```python
from build123d import *

# Parameters (mm, degrees)
SKETCH1_W               = 50.8
SKETCH1_H               = 50.8
BOSS_EXTRUDE1_DEPTH     = 19.05
F_1_4_CLEARANCE_HOLE1_D = 6.7564
SKETCH9_W               = 12.7
SKETCH9_H               = 50.8
SKETCH9_W_2             = 50.8
SKETCH9_H_2             = 12.7
SKETCH9_W_3             = 31.75
SKETCH9_H_3             = 31.75
CUT_EXTRUDE1_DEPTH      = 12.7


with BuildPart() as part:
    # Sketch1 → Boss-Extrude1 (new body)
    with BuildSketch(Plane(origin=(0, 0, 0), x_dir=(1, 0, 0), z_dir=(0, 1, 0))):
        Rectangle(SKETCH1_W, SKETCH1_H)
    extrude(amount=BOSS_EXTRUDE1_DEPTH)

    # 1/4 Clearance Hole1 (through all)
    with Locations(Plane(origin=(0, 19.05, 0), x_dir=(1, 0, 0), z_dir=(0, 1, 0))):
        with Locations((-19.05, 19.05), (19.05, 19.05), (19.05, -19.05), (-19.05, -19.05)):
            Hole(F_1_4_CLEARANCE_HOLE1_D / 2)

    # Sketch9 → Cut-Extrude1 (cut)
    with BuildSketch(Plane.XZ):
        Rectangle(SKETCH9_W, SKETCH9_H)
        Rectangle(SKETCH9_W_2, SKETCH9_H_2)
        Rectangle(SKETCH9_W_3, SKETCH9_H_3)
    extrude(amount=-CUT_EXTRUDE1_DEPTH, mode=Mode.SUBTRACT)


solid = part.part
```
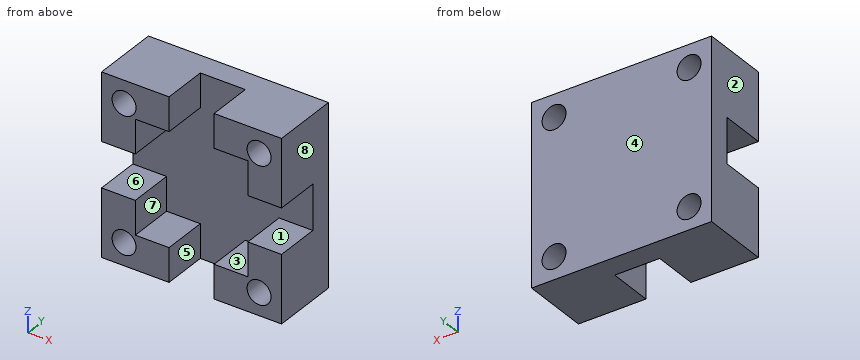
Source: CAD feature listing. Evaluate the final solid. Frame: model axes, mm. Face numbers are marked on the shaded views. A direction names the side the tool comes from. Coordinates: 2 decimals unless noted, no trailing zeros. Write each loop counter-clockwise with the first axis right and the second up, starting at its lowest first coordinate (ties: lowest second). Pieces come first, ordered by that corner, then holes. Notation, with made-up numbers: (16, 86.25) -> (72, 86.25) arc R33 ccw to (72, 117.25) -> close; hole circle Ø11 at (55.5, -7.5). An arc over 180 degrees is marked (long way). Return JSON: item names as keys, results as strings. Group by question number.
1) Ray query, line 1 along X through (y, z) = (10.25, -19.05); line 2 along X through (y, z) = (15, -19.05). Return the intervals inside material, ascending.
2) Section query D-D, the plane z = 8.5. Return loops of the section in (x, y) (3 decimals).
3) Section query C-C, the plane x = -19.05. Return loops of the section in (y, z), plus the area to 3 significant figures.
4) Set-up query: the marked faces 1, 2, 3, 4 and 5. Return all of +Z, -Z, +X, -X, +Y, -Y with unobstructed straight access to the full face (end or side cutting, diameter ignored); none if empty.
5) Section query A-A, the plane y = 7. Return loops of the section in (x, z) (3 decimals), plus the area to 3 significant figures.
6) Contact query for a flat-ended pin moving along its axis: P1, Ø3, axis at x = 16.5, z = 0, coming from the -Y side. Output: stop coordinate, or through.
7) Section query B-B, the plane z = 19.05. Return loops of the section in (x, y).
8) Mould query, pull axis X, two halves, no side actions, for the marked faces 6, 7 and 8. Classes: +X half, -X half, draft (parallel to the pull), parting line (faces both ways), or undercut.
From the geometry:
{
 "1": {"line 1": "-25.4 to -22.43, -15.67 to -6.35, 6.35 to 15.67, 22.43 to 25.4", "line 2": "-25.4 to -22.43, -15.67 to 15.67, 22.43 to 25.4"},
 "2": {"outline": "(-25.4, 0) -> (-15.875, 0) -> (-15.875, 12.7) -> (15.875, 12.7) -> (15.875, 0) -> (25.4, 0) -> (25.4, 19.05) -> (-25.4, 19.05) -> close"},
 "3": {"outline": "(0, -25.4) -> (19.05, -25.4) -> (19.05, -22.43) -> (0, -22.43) -> close; (0, -15.67) -> (19.05, -15.67) -> (19.05, 15.67) -> (0, 15.67) -> (0, 6.35) -> (12.7, 6.35) -> (12.7, -6.35) -> (0, -6.35) -> close; (0, 22.43) -> (19.05, 22.43) -> (19.05, 25.4) -> (0, 25.4) -> close", "area": "549 mm²"},
 "4": {"face 1": "+X, -X, -Y", "face 2": "+Z, -Z, -X, +Y, -Y", "face 3": "-Y", "face 4": "+Z, -Z, +X, -X, +Y", "face 5": "+Z, -Z, -Y"},
 "5": {"outline": "(-25.4, -25.4) -> (-6.35, -25.4) -> (-6.35, -15.875) -> (-15.875, -15.875) -> (-15.875, -6.35) -> (-25.4, -6.35) -> close; (-25.4, 6.35) -> (-15.875, 6.35) -> (-15.875, 15.875) -> (-6.35, 15.875) -> (-6.35, 25.4) -> (-25.4, 25.4) -> close; (6.35, -25.4) -> (25.4, -25.4) -> (25.4, -6.35) -> (15.875, -6.35) -> (15.875, -15.875) -> (6.35, -15.875) -> close; (6.35, 15.875) -> (15.875, 15.875) -> (15.875, 6.35) -> (25.4, 6.35) -> (25.4, 25.4) -> (6.35, 25.4) -> close; hole circle Ø6.756 at (-19.05, -19.05); hole circle Ø6.756 at (-19.05, 19.05); hole circle Ø6.756 at (19.05, -19.05); hole circle Ø6.756 at (19.05, 19.05)", "area": "945 mm²"},
 "6": {"P1": "y = 12.7"},
 "7": {"outline": "(-25.4, 0) -> (-22.43, 0) -> (-22.43, 19.05) -> (-25.4, 19.05) -> close; (-15.67, 0) -> (-6.35, 0) -> (-6.35, 12.7) -> (6.35, 12.7) -> (6.35, 0) -> (15.67, 0) -> (15.67, 19.05) -> (-15.67, 19.05) -> close; (22.43, 0) -> (25.4, 0) -> (25.4, 19.05) -> (22.43, 19.05) -> close"},
 "8": {"face 6": "draft", "face 7": "undercut", "face 8": "+X half"}
}
